Check sheet for the modelled part. Datum: model origin and axes. Units: mm. A direction names the side the tool comes from. Round coordinates to 2 decimals unless told otherwise and drop trailing zeros. Loops run counter-clockwise (first coordinate to the right, second up) from the corner with the lowest first, then second, coordinate; pieces in that order, holes last. Notation, with made-up numbers: (65.5, 40) - (84.5, 40) arc R24 cw to (84.5, 52) - close; hole circle Ø8 at (7, 54.25). An arc over 180 degrees is marked (long way). Put each result on its own line as item: value.
```python
from build123d import *

# Parameters (mm, degrees)
SKETCH1_R                = 1
BOSS_EXTRUDE1_DEPTH      = 1.5
BOSS_EXTRUDE2_DEPTH      = 2.5
BOSS_EXTRUDE3_DEPTH      = 60
BOSS_EXTRUDE3_DEPTH_BACK = 40
SKETCH4_W                = 5
SKETCH4_H                = 50


with BuildPart() as part:
    # Sketch1 → Boss-Extrude1 (new, symmetric)
    with BuildSketch(Plane(origin=(0, 0, 0), x_dir=(1, 0, 0), z_dir=(0, 1, 0))):
        with BuildLine():
            Line((5, 77.5), (-35, 77.5))
            Line((-35, 77.5), (-35, 44))
            Line((-35, 44), (-20, 24))
            Line((-20, 24), (-20, 0))
            ThreePointArc((-20, 0), (0, -20), (20, 0))
            Line((20, 0), (20, 24))
            Line((20, 24), (5, 44))
            Line((5, 44), (5, 77.5))
        make_face()
        with Locations(Location((0, 7.5, 0), (0, 0, 270))):
            Circle(SKETCH1_R, mode=Mode.SUBTRACT)
        with Locations(Location((0, 10.5, 0), (0, 0, 270))):
            Circle(SKETCH1_R, mode=Mode.SUBTRACT)
        with Locations(Location((0, 13.5, 0), (0, 0, 270))):
            Circle(SKETCH1_R, mode=Mode.SUBTRACT)
        with Locations(Location((11.691342951, 6.75, 0), (0, 0, 270))):
            Circle(SKETCH1_R, mode=Mode.SUBTRACT)
        with Locations(Location((6.495190528, 3.75, 0), (0, 0, 270))):
            Circle(SKETCH1_R, mode=Mode.SUBTRACT)
        with Locations(Location((9.09326674, 5.25, 0), (0, 0, 270))):
            Circle(SKETCH1_R, mode=Mode.SUBTRACT)
        with Locations(Location((11.691342951, -6.75, 0), (0, 0, 270))):
            Circle(SKETCH1_R, mode=Mode.SUBTRACT)
        with Locations(Location((6.495190528, -3.75, 0), (0, 0, 270))):
            Circle(SKETCH1_R, mode=Mode.SUBTRACT)
        with Locations(Location((9.09326674, -5.25, 0), (0, 0, 270))):
            Circle(SKETCH1_R, mode=Mode.SUBTRACT)
        with Locations(Location((0, -13.5, 0), (0, 0, 270))):
            Circle(SKETCH1_R, mode=Mode.SUBTRACT)
        with Locations(Location((0, -7.5, 0), (0, 0, 270))):
            Circle(SKETCH1_R, mode=Mode.SUBTRACT)
        with Locations(Location((0, -10.5, 0), (0, 0, 270))):
            Circle(SKETCH1_R, mode=Mode.SUBTRACT)
        with Locations(Location((-11.691342951, -6.75, 0), (0, 0, 270))):
            Circle(SKETCH1_R, mode=Mode.SUBTRACT)
        with Locations(Location((-6.495190528, -3.75, 0), (0, 0, 270))):
            Circle(SKETCH1_R, mode=Mode.SUBTRACT)
        with Locations(Location((-9.09326674, -5.25, 0), (0, 0, 270))):
            Circle(SKETCH1_R, mode=Mode.SUBTRACT)
        with Locations(Location((-11.691342951, 6.75, 0), (0, 0, 270))):
            Circle(SKETCH1_R, mode=Mode.SUBTRACT)
        with Locations(Location((-6.495190528, 3.75, 0), (0, 0, 270))):
            Circle(SKETCH1_R, mode=Mode.SUBTRACT)
        with Locations(Location((-9.09326674, 5.25, 0), (0, 0, 270))):
            Circle(SKETCH1_R, mode=Mode.SUBTRACT)
    extrude(amount=BOSS_EXTRUDE1_DEPTH, both=True)

    # Sketch3 → Boss-Extrude2 (add, symmetric)
    with BuildSketch(Plane(origin=(-15, 0, 0), x_dir=(0, 0, -1), z_dir=(1, 0, 0))):
        Polygon((60.75, 1.5), (77.5, 9), (77.5, 1.5), align=None)
    boss_extrude2 = extrude(amount=BOSS_EXTRUDE2_DEPTH, both=True)

    # Mirror1: Boss-Extrude2 across plane
    add(boss_extrude2.mirror(Plane.ZX))

    # Sketch4 → Boss-Extrude3 (add, two sides: drawn at the far end of the back side and taken through both)
    with BuildSketch(Plane(origin=(-15, 0, 0), x_dir=(0, 0, -1), z_dir=(1, 0, 0)).offset(-BOSS_EXTRUDE3_DEPTH_BACK)):
        with Locations((80, 0)):
            Rectangle(SKETCH4_W, SKETCH4_H)
    extrude(amount=BOSS_EXTRUDE3_DEPTH + BOSS_EXTRUDE3_DEPTH_BACK)


solid = part.part
```
Item 1: Go/stop test with flat-tipped pins: pin 1 (2.5 mm diameter, centred on x = 11.69, z = -6.75, fed in from +Y); pin 2 (0.9 mm diameter, centred on y = 0.5, z = -7, fed in from +X); pin 3 (2.5 mm diameter, centred on y = 0, z = -66.5, fed in from -X). Record where each tip stops, or that it passes through.
Filled sheet:
pin 1: y = 1.5
pin 2: x = 20
pin 3: x = -35
Item 2: Release check for a two-part mould opening along Z. For faces 1 (the flat face through (-6, 0, -82.5)), 2 (the flat face through (-12.5, -4, -73)), 3 (the flat face through (-14.96, 5.2, -69.01)), 4 (the flat face through (5, 0, -61)) record: +Z half, -Z half, draft (parallel to the pull), parting line (faces both ways), or undercut.
Filled sheet:
face 1: -Z half
face 2: draft
face 3: +Z half
face 4: undercut
Item 3: Section check C-C on z = -19. Enter the section's corners in (x, y), then the cut area to 3 significant figures.
Filled sheet:
outline: (-20, -1.5) - (20, -1.5) - (20, 1.5) - (-20, 1.5) - close
area: 120 mm²
Item 4: Section check A-A on y = -4.5. Enter the section's corners in (x, z), then the cut area to 3 significant figures.
Filled sheet:
outline: (-55, -82.5) - (45, -82.5) - (45, -77.5) - (-12.5, -77.5) - (-12.5, -67.45) - (-17.5, -67.45) - (-17.5, -77.5) - (-55, -77.5) - close
area: 550 mm²
Item 5: Section check D-D on x = 28. Enter the section's corners in (y, z).
Filled sheet:
outline: (-25, -82.5) - (25, -82.5) - (25, -77.5) - (-25, -77.5) - close
Item 6: Tool access check on faces 5 (the flat face through (-17.5, -4, -73)), 6 (the flat face through (-12.5, 4, -73)), 7 (the flat face through (-20, 0, -12)). Record the directions out of +Z, -Z, +X, -X, +Y, -Y that give a thin tool (end or side, any length) a straight path to the whole face; none if there is none.
Filled sheet:
face 5: +Z, -X, -Y
face 6: +Z, +X, +Y
face 7: +Z, -X, +Y, -Y
Item 7: Section check B-B on x = -33.5. Enter the section's corners in (y, z).
Filled sheet:
outline: (-25, -82.5) - (25, -82.5) - (25, -77.5) - (1.5, -77.5) - (1.5, -42) - (-1.5, -42) - (-1.5, -77.5) - (-25, -77.5) - close
Item 8: Thickness scan on line 1 (X direction, y = 0.1, z = -3.75); line 2 (Z direction, x = 29, y = -20); line 3 (Y direction, x = 14.5, z = -31). Record the ranges inside material, lowest first. Write a range as from..to.
Filled sheet:
line 1: -20..-7.5, -5.5..5.5, 7.5..20
line 2: -82.5..-77.5
line 3: -1.5..1.5
